Print and shaded views of the part. All mm, measured from the part's lowest x, y and z. A direction names the side the tool comes from. Coordinates: 2 decimals unless noted, no trailing zeros. Order: outer loops, then holes, each group sorted by start corner. A loop starts at its lowest first (then second) coordinate and runs counter-clockwise, first axis right, second up. Notation, with made-up numbers: M -37,55.25 L 8,55.25 A22 cw 8,80.25 Z; hole C -25,83 d4. An arc over 180 degrees is marked long. Return JSON: item names as keys, results as strings.
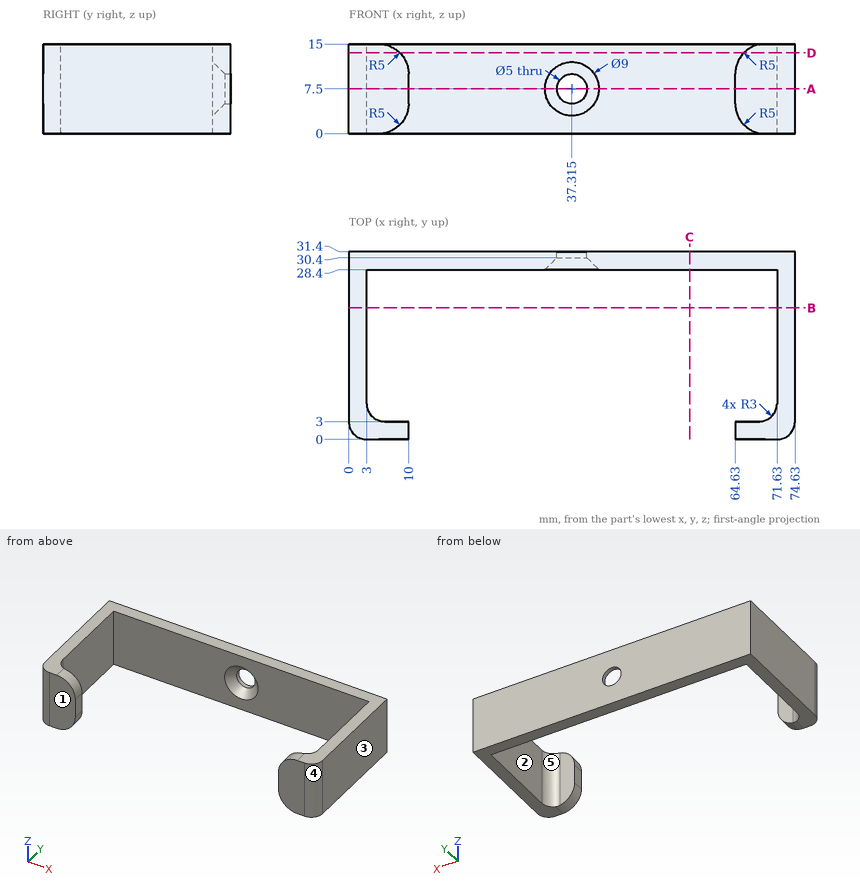
Item 1: 3-axis set-ups, long thin cutter, end or side, ignore diameter. For the marked faces 4 and 5: which of +Z, -Z, +X, -X, +Y, -Y reach the whole face in a straight line?
Check result:
{"face 4": "+Z, -Z, +X, -Y", "face 5": "+Z, -Z"}
Item 2: Pull direction X, two halves, no side cores. Call the marked faces 1, 2 and 3: +X half, -X half, draft (parallel to the pull), parting line (faces both ways), or undercut.
Check result:
{"face 1": "draft", "face 2": "undercut", "face 3": "+X half"}
Item 3: Saw through at B-B (y = 22). Write the cut outline in (x, z).
Check result:
{"outline": "M 0,0 L 3,0 L 3,15 L 0,15 Z; M 71.63,0 L 74.63,0 L 74.63,15 L 71.63,15 Z"}
Item 4: Wall check: line 1 (X direction, y = 20.5, z = 3.25); line 2 (Y direction, x = 27.5, z = 2.5); line 3 (Y direction, x = 9, z = 7). Give the ranges that are in metal, low to high.
Check result:
{"line 1": "x = 0 to 3, 71.63 to 74.63", "line 2": "y = 28.4 to 31.4", "line 3": "y = 0 to 3, 28.4 to 31.4"}
Item 5: Saw through at A-A (z = 7.5). Write the cut outline in (x, y) (3 decimals), and give its area (3 significant figures).
Check result:
{"outline": "M 0,3 A3 ccw 3,0 L 10,0 L 10,3 L 6,3 A3 cw 3,6 L 3,28.4 L 32.815,28.4 L 34.815,30.4 L 34.815,31.4 L 0,31.4 Z; M 39.815,30.4 L 41.815,28.4 L 71.63,28.4 L 71.63,6 A3 cw 68.63,3 L 64.63,3 L 64.63,0 L 71.63,0 A3 ccw 74.63,3 L 74.63,31.4 L 39.815,31.4 Z", "area": "417 mm2"}
Item 6: Saw through at C-C (x = 57). Write the cut outline in (y, z).
Check result:
{"outline": "M 28.4,0 L 31.4,0 L 31.4,15 L 28.4,15 Z"}
Item 7: Drop flat-ended pins along their axis: pin 1 Ø0.9 at (y, z) = (2, 7) entering from +X; pin 2 Ø0.9 at (y, z) = (1, 7.5) entering from -X; pin 3 Ø1.5 at (x, z) = (34.5, 5.5) entering from -Y. Give the stop position or say it passes through.
Check result:
{"pin 1": "stops at x = 74.58", "pin 2": "stops at x = 0.43", "pin 3": "stops at y = 28.7"}
Item 8: Saw through at D-D (z = 13.5). Write the cut outline in (x, y), and give its area (3 significant figures).
Check result:
{"outline": "M 0,3 A3 ccw 3,0 L 8.57,0 L 8.57,3 L 6,3 A3 cw 3,6 L 3,28.4 L 71.63,28.4 L 71.63,6 A3 cw 68.63,3 L 66.06,3 L 66.06,0 L 71.63,0 A3 ccw 74.63,3 L 74.63,31.4 L 0,31.4 Z", "area": "428 mm2"}
